Geometry: final body of the model. Coordinates: model frame, mm. Coordinates: 2 decimals unless noted, no trailing zeros. Order: outer loops, then holes, each group sorted by start corner. A loop starts at its lowest first (then second) coordinate and runs counter-clockwise, first axis right, second up. Notation, with made-up numbers: (76, -12.5) -> (131, -12.5) arc R23 cw to (131, 14.5) -> close; hole circle Ø10 at (-11, 82.25). An arc over 180 degrees is marked (long way). Use one line per item in the form item = value.
```python
from build123d import *

# Parameters (mm, degrees)
SKETCH_1_W        = 22.5
SKETCH_1_H        = 14
EXTRUDE_1_DEPTH   = 7.2
SKETCH_2_R        = 0.25
EXTRUDE_2_DEPTH   = 6.3
SKETCH_3_W        = 1.121019108
SKETCH_3_H        = 1.732484076
EXTRUDE_1_2_DEPTH = 0.01


with BuildPart() as part:
    # 草图1 → Extrude 1 (new body)
    with BuildSketch(Plane(origin=(0, 0, 0), x_dir=(1, 0, 0), z_dir=(0, 1, 0))):
        Rectangle(SKETCH_1_W, SKETCH_1_H)
    extrude(amount=EXTRUDE_1_DEPTH)

    # 草图2 → 拉伸2 (add)
    with BuildSketch(Plane.XZ):
        with Locations(Location((6.224686657, 4.1, 0), (0, 0, 90))):
            Circle(SKETCH_2_R)
        with Locations(Location((3.734811994, 4.1, 0), (0, 0, 90))):
            Circle(SKETCH_2_R)
        with Locations(Location((1.244937331, 4.1, 0), (0, 0, 90))):
            Circle(SKETCH_2_R)
        with Locations(Location((-1.244937331, 4.1, 0), (0, 0, 90))):
            Circle(SKETCH_2_R)
        with Locations(Location((-3.734811994, 4.1, 0), (0, 0, 90))):
            Circle(SKETCH_2_R)
        with Locations(Location((-6.224686657, 4.1, 0), (0, 0, 90))):
            Circle(SKETCH_2_R)
        with Locations(Location((-6.224686657, -4.1, 0), (0, 0, 90))):
            Circle(SKETCH_2_R)
        with Locations(Location((-3.734811994, -4.1, 0), (0, 0, 90))):
            Circle(SKETCH_2_R)
        with Locations(Location((-1.244937331, -4.1, 0), (0, 0, 90))):
            Circle(SKETCH_2_R)
        with Locations(Location((1.244937331, -4.1, 0), (0, 0, 90))):
            Circle(SKETCH_2_R)
        with Locations(Location((3.734811994, -4.1, 0), (0, 0, 90))):
            Circle(SKETCH_2_R)
        with Locations(Location((6.224686657, -4.1, 0), (0, 0, 90))):
            Circle(SKETCH_2_R)
    extrude(amount=EXTRUDE_2_DEPTH)

    # 草图3 → Extrude 1 2 (add)
    with BuildSketch(Plane(origin=(0, 7.2, 0), x_dir=(1, 0, 0), z_dir=(0, 1, 0))):
        Polygon((-4.991082803, 0.076433121), (-6.112101911, 0.633757962), (-6.112101911, 2.813694268), (-5.556369427, 3.286624204), (-4.991082803, 2.813694268), align=None)
        Polygon((-5.737898089, 3.377388535), (-6.311146497, 2.929936306), (-9.034076433, 2.929936306), (-9.553184713, 3.377388535), (-9.034076433, 3.847133758), (-6.311146497, 3.847133758), align=None)
        Polygon((-4.991082803, -2.910828025), (-5.556369427, -3.388535032), (-6.112101911, -2.910828025), (-6.112101911, -0.632165605), (-4.991082803, -0.159235669), align=None)
        Polygon((-5.223566879, -0.035031847), (-6.242675159, -0.464968153), (-9.002229299, -0.484076433), (-10.038853503, -0.020700637), (-9.008598726, 0.484076433), (-6.268152866, 0.484076433), align=None)
        Polygon((-9.169426752, 0.633757962), (-10.29044586, 0.082802548), (-10.29044586, 2.813694268), (-9.734713376, 3.286624204), (-9.169426752, 2.813694268), align=None)
        Polygon((-9.169426752, -2.888535032), (-9.734713376, -3.361464968), (-10.29044586, -2.888535032), (-10.29044586, -0.127388535), (-9.169426752, -0.632165605), align=None)
        Polygon((-5.737898089, -3.530254777), (-6.311146497, -4), (-9.034076433, -4), (-9.553184713, -3.530254777), (-9.034076433, -3.082802548), (-6.311146497, -3.082802548), align=None)
        with Locations((-4.084076433, -3.133757962)):
            Rectangle(SKETCH_3_W, SKETCH_3_H)
        Polygon((2.020382166, 0.076433121), (0.899363057, 0.633757962), (0.899363057, 2.813694268), (1.455095541, 3.286624204), (2.020382166, 2.813694268), align=None)
        Polygon((1.273566879, 3.377388535), (0.700318471, 2.929936306), (-2.022611465, 2.929936306), (-2.541719745, 3.377388535), (-2.022611465, 3.847133758), (0.700318471, 3.847133758), align=None)
        Polygon((2.020382166, -2.910828025), (1.455095541, -3.388535032), (0.899363057, -2.910828025), (0.899363057, -0.632165605), (2.020382166, -0.159235669), align=None)
        Polygon((1.787898089, -0.035031847), (0.768789809, -0.464968153), (-1.990764331, -0.484076433), (-3.027388535, -0.020700637), (-1.997133758, 0.484076433), (0.743312102, 0.484076433), align=None)
        Polygon((-2.157961783, 0.633757962), (-3.278980892, 0.082802548), (-3.278980892, 2.813694268), (-2.723248408, 3.286624204), (-2.157961783, 2.813694268), align=None)
        Polygon((-2.157961783, -2.888535032), (-2.723248408, -3.361464968), (-3.278980892, -2.888535032), (-3.278980892, -0.127388535), (-2.157961783, -0.632165605), align=None)
        Polygon((1.273566879, -3.530254777), (0.700318471, -4), (-2.022611465, -4), (-2.541719745, -3.530254777), (-2.022611465, -3.082802548), (0.700318471, -3.082802548), align=None)
        with Locations((2.927388535, -3.133757962)):
            Rectangle(SKETCH_3_W, SKETCH_3_H)
        Polygon((9.031847134, 0.076433121), (7.910828025, 0.633757962), (7.910828025, 2.813694268), (8.46656051, 3.286624204), (9.031847134, 2.813694268), align=None)
        Polygon((8.285031847, 3.377388535), (7.711783439, 2.929936306), (4.988853503, 2.929936306), (4.469745223, 3.377388535), (4.988853503, 3.847133758), (7.711783439, 3.847133758), align=None)
        Polygon((9.031847134, -2.910828025), (8.46656051, -3.388535032), (7.910828025, -2.910828025), (7.910828025, -0.632165605), (9.031847134, -0.159235669), align=None)
        Polygon((8.799363057, -0.035031847), (7.780254777, -0.464968153), (5.020700637, -0.484076433), (3.984076433, -0.020700637), (5.01433121, 0.484076433), (7.75477707, 0.484076433), align=None)
        Polygon((4.853503185, 0.633757962), (3.732484076, 0.082802548), (3.732484076, 2.813694268), (4.288216561, 3.286624204), (4.853503185, 2.813694268), align=None)
        Polygon((4.853503185, -2.888535032), (4.288216561, -3.361464968), (3.732484076, -2.888535032), (3.732484076, -0.127388535), (4.853503185, -0.632165605), align=None)
        Polygon((8.285031847, -3.530254777), (7.711783439, -4), (4.988853503, -4), (4.469745223, -3.530254777), (4.988853503, -3.082802548), (7.711783439, -3.082802548), align=None)
        with Locations((9.938853503, -3.133757962)):
            Rectangle(SKETCH_3_W, SKETCH_3_H)
    extrude(amount=EXTRUDE_1_2_DEPTH)


solid = part.part
```
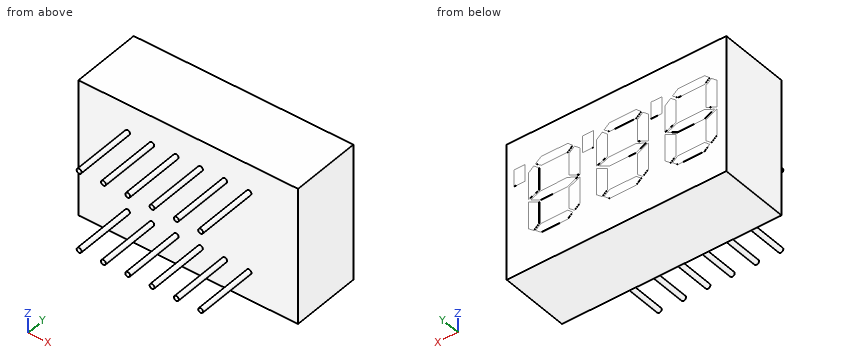
1) Section C-C, the plane y = -3. Give the number of separate pieces and of enclosed holes in the cut face, and give its area (3 significant figures).
Results found:
separate_pieces = 12
enclosed_holes = 0
area = 2.36 mm2
2) Section D-D, the plane z = -4.1. Output: boundary loops of the cut face in (x, y).
Results found:
outline = (-11.25, 0) -> (-6.47, 0) -> (-6.47, -6.3) -> (-5.97, -6.3) -> (-5.97, 0) -> (-3.98, 0) -> (-3.98, -6.3) -> (-3.48, -6.3) -> (-3.48, 0) -> (-1.49, 0) -> (-1.49, -6.3) -> (-0.99, -6.3) -> (-0.99, 0) -> (0.99, 0) -> (0.99, -6.3) -> (1.49, -6.3) -> (1.49, 0) -> (3.48, 0) -> (3.48, -6.3) -> (3.98, -6.3) -> (3.98, 0) -> (5.97, 0) -> (5.97, -6.3) -> (6.47, -6.3) -> (6.47, 0) -> (11.25, 0) -> (11.25, 7.2) -> (-11.25, 7.2) -> close
3) Contact query for flat-ended pins moving along their axis: P1, Ø3, axis at x = 0, z = -5.5, coming from the -Y side; P2, Ø2, axis at y = -2.5, z = -5, coming from the +X side. Output: stop coordinate, or through.
Results found:
P1 = 0
P2 = 6.47
4) Material intervals for probe 1 along X at (y, z) = (-2, -4); probe 2 along Y at (x, z) = (3.5, 1), sorted ascending. Write a range as from..to.
Results found:
probe_1 = -6.45..-6, -3.96..-3.51, -1.47..-1.02, 1.02..1.47, 3.51..3.96, 6..6.45
probe_2 = 0..7.2
